Design review of the part built by this model. Coordinates are the model's own, in mm. A direction names the side the tool comes from. Coordinates: 2 decimals unless noted, no trailing zeros. Order: outer loops, then holes, each group sorted by start corner. A loop starts at its lowest first (then second) coordinate and runs counter-clockwise, first axis right, second up. Notation, with made-up numbers: (8, -3.75) -> (12, -3.75) arc R15 ccw to (12, 16.25) -> close; hole circle Ø7 at (22, -19). An arc over 180 degrees is marked (long way). Use a Markdown table: item, result. Add a question column.
Q1. Add section B-B (y = 18.75). State the section outline as (x, z) points, then the cut area to 3 significant figures.
Q2. The part is to be moulded in two halves that separate along Z. For faces 1 (the face through (14.143, 2.028, -21.247)), 2 (the face through (-13.02, 2.03, -14.9)), 3 (the face through (0, 2, -30)), 4 (the face through (0, 4, -19)), say which applies: pulls with the +Z half, pulls with the -Z half, needs draft (parallel to the pull), parting line crosses it, or undercut.
Q3. Add section D-D (z = -12.5). State the section outline as (x, y) points, then the cut area to 3 significant figures.
Q4. Add section A-A (x = -10). State the section outline as (y, z) points.
Q5. Wall thickness on probe 1 along X at (y, z) = (1.35, -18); probe 2 along X at (y, z) = (22, -2.25); probe 3 along Z at (x, y) = (9.5, 16): over which ranges is each line inside the solid? List them lowest first.
Q6. Add section C-C (z = -18). State the section outline as (x, y) points, then the cut area to 3 significant figures.
Q7. Machinability: for faces 5 (the face through (-0.28, 2.406, -2.281)), 6 (the face through (0, 19, -4)), which of the approach directions +Z, -Z, +X, -X, +Y, -Y give a long, thin tool a straight path to every point of the face, cutting with its end or side? Answer none if there is none.
Q8. Insertion check: pin 1 (5 mm diameter, centred on x = 10, y = 20, fed in from +Z) (1 decimal); pin 2 (8 mm diameter, centred on x = -0.5, y = 26.5, fed in from -Z); pin 3 (6.5 mm diameter, centred on x = -1.5, z = -22.5, fed in from +Y). Each pin has a flat end and moves straight along its axis. Give the tip position at first contact, or say it passes through.
from build123d import *

# Parameters (mm, degrees)
EXTRUDE_1_DEPTH      = 20
EXTRUDE_1_DEPTH_BACK = 20
CUT_EXTRUDE_1_DEPTH  = 4
CUT_EXTRUDE_2_DEPTH  = 4
SKETCH_4_W           = 3.25
SKETCH_4_H           = 9
SKETCH_5_W           = 3.25
SKETCH_5_H           = 9
SKETCH_6_W           = 3.25
SKETCH_6_H           = 9
SKETCH_7_W           = 3.25
SKETCH_7_H           = 9


with BuildPart() as part:
    # Sketch 1 → Extrude 1 (new, two sides: drawn at the far end of the back side and taken through both)
    with BuildSketch(Plane(origin=(0, 0, 0), x_dir=(0, 0, -1), z_dir=(1, 0, 0)).offset(-EXTRUDE_1_DEPTH_BACK)):
        with BuildLine():
            Line((8, 0), (30, 0))
            Line((30, 0), (30, 4))
            Line((30, 4), (8, 4))
            ThreePointArc((8, 4), (5.171572875, 5.171572875), (4, 8))
            Line((4, 8), (4, 30))
            Line((4, 30), (0, 30))
            Line((0, 30), (0, 8))
            ThreePointArc((0, 8), (2.343145751, 2.343145751), (8, 0))
        make_face()
    extrude(amount=EXTRUDE_1_DEPTH + EXTRUDE_1_DEPTH_BACK)

    # Sketch 2 → Cut-Extrude 1 (cut)
    with BuildSketch(Plane.XY):
        Polygon((-22, 32), (-22, 27), (-20, 27), (-20, 28), (-18, 30), (18, 30), (20, 28), (20, 27), (22, 27), (22, 32), align=None)
    extrude(amount=-CUT_EXTRUDE_1_DEPTH, mode=Mode.SUBTRACT)

    # Sketch 3 → Cut-Extrude 2 (cut)
    with BuildSketch(Plane(origin=(0, 0, 0), x_dir=(1, 0, 0), z_dir=(0, 1, 0))):
        Polygon((-22, 32), (-22, 27), (-20, 27), (-20, 28), (-18, 30), (18, 30), (20, 28), (20, 27), (22, 27), (22, 32), align=None)
    extrude(amount=CUT_EXTRUDE_2_DEPTH, mode=Mode.SUBTRACT)

    # Sketch 4 → Cut-Revolve 1 (revolve, cut)
    with BuildSketch(Plane(origin=(0, 20, 0), x_dir=(1, 0, 0), z_dir=(0, 1, 0)), mode=Mode.PRIVATE) as cut_revolve_1_sk:
        with Locations((11.625, 4.5)):
            Rectangle(SKETCH_4_W, SKETCH_4_H)
    revolve(cut_revolve_1_sk.sketch.rotate(Axis((10, 20, 0), (0, 0, -1)), 180), axis=Axis((10, 20, 0), (0, 0, -1)), mode=Mode.SUBTRACT)

    # Sketch 5 → Cut-Revolve 2 (revolve, cut)
    with BuildSketch(Plane(origin=(0, 20, 0), x_dir=(1, 0, 0), z_dir=(0, 1, 0)), mode=Mode.PRIVATE) as cut_revolve_2_sk:
        with Locations((-8.375, 4.5)):
            Rectangle(SKETCH_5_W, SKETCH_5_H)
    revolve(cut_revolve_2_sk.sketch.rotate(Axis((-10, 20, 0), (0, 0, -1)), 180), axis=Axis((-10, 20, 0), (0, 0, -1)), mode=Mode.SUBTRACT)

    # Sketch 6 → Cut-Revolve 3 (revolve, cut)
    with BuildSketch(Plane.XY.offset(-18), mode=Mode.PRIVATE) as cut_revolve_3_sk:
        with Locations((15.625, 4.5)):
            Rectangle(SKETCH_6_W, SKETCH_6_H)
    revolve(cut_revolve_3_sk.sketch.rotate(Axis((14, 0, -18), (0, 1, 0)), 270), axis=Axis((14, 0, -18), (0, 1, 0)), mode=Mode.SUBTRACT)

    # Sketch 7 → Cut-Revolve 4 (revolve, cut)
    with BuildSketch(Plane.XY.offset(-18), mode=Mode.PRIVATE) as cut_revolve_4_sk:
        with Locations((-12.375, 4.5)):
            Rectangle(SKETCH_7_W, SKETCH_7_H)
    revolve(cut_revolve_4_sk.sketch.rotate(Axis((-14, 0, -18), (0, 1, 0)), 270), axis=Axis((-14, 0, -18), (0, 1, 0)), mode=Mode.SUBTRACT)


solid = part.part
Established:
| question | item | result |
|---|---|---|
| 1 | outline | (-20, -4) -> (-13, -4) -> (-13, 0) -> (-20, 0) -> close; (-7, -4) -> (7, -4) -> (7, 0) -> (-7, 0) -> close; (13, -4) -> (20, -4) -> (20, 0) -> (13, 0) -> close |
| 1 | area | 112 mm^2 |
| 2 | face 1 | undercut |
| 2 | face 2 | undercut |
| 2 | face 3 | pulls with the -Z half |
| 2 | face 4 | needs draft |
| 3 | outline | (-20, 0) -> (20, 0) -> (20, 4) -> (-20, 4) -> close |
| 3 | area | 160 mm^2 |
| 4 | outline | (0, -30) -> (4, -30) -> (4, -8) arc R4 cw to (8, -4) -> (16.75, -4) -> (16.75, 0) -> (8, 0) arc R8 ccw to (0, -8) -> close; (23.25, -4) -> (30, -4) -> (30, 0) -> (23.25, 0) -> close |
| 5 | probe 1 | -20 to -17.25, -10.75 to 10.75, 17.25 to 20 |
| 5 | probe 2 | -20 to -12.56, -7.44 to 7.44, 12.56 to 20 |
| 5 | probe 3 | -4 to 0 |
| 6 | outline | (-20, 0) -> (-17.25, 0) -> (-17.25, 4) -> (-20, 4) -> close; (-10.75, 0) -> (10.75, 0) -> (10.75, 4) -> (-10.75, 4) -> close; (17.25, 0) -> (20, 0) -> (20, 4) -> (17.25, 4) -> close |
| 6 | area | 108 mm^2 |
| 7 | face 5 | +Z, +X, -X, -Y |
| 7 | face 6 | -Z, +X, -X, +Y |
| 8 | pin 1 | through |
| 8 | pin 2 | z = -4 |
| 8 | pin 3 | y = 4 |
